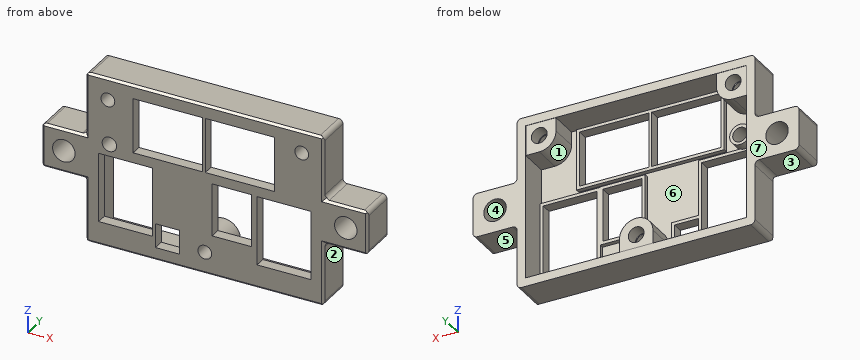
```python
from build123d import *

# Parameters (mm, degrees)
SKETCH1_W           = 54
SKETCH1_H           = 39
SKETCH1_W_2         = 10
SKETCH1_H_2         = 10
SKETCH1_R           = 2.5527
BOSS_EXTRUDE1_DEPTH = 8
SKETCH2_W           = 50.1
SKETCH2_H           = 35.1
CUT_EXTRUDE1_DEPTH  = 0.0762
CUT_EXTRUDE2_DEPTH  = 6.5
SKETCH4_R           = 1.56
CUT_EXTRUDE3_DEPTH  = 43.568023286
SKETCH5_R           = 1.79
CUT_EXTRUDE4_DEPTH  = 2.92
SKETCH6_W           = 12.25
SKETCH6_H           = 15.75
SKETCH6_W_2         = 15.75
SKETCH6_H_2         = 12.5
SKETCH6_W_3         = 5.5
SKETCH6_H_3         = 5.5
CUT_EXTRUDE5_DEPTH  = 43.337883821
SKETCH7_W           = 8.9
SKETCH7_H           = 12
CUT_EXTRUDE6_DEPTH  = 43.337883821
CHAMFER1_SIZE       = 0.5
SKETCH9_R           = 1.651
CUT_EXTRUDE8_DEPTH  = 43.337883821
BOSS_EXTRUDE2_START = 3
SKETCH10_R          = 2.3375
SKETCH10_R_2        = 1.651
BOSS_EXTRUDE2_DEPTH = 3
SKETCH11_W          = 5.5
SKETCH11_H          = 5.5
SKETCH11_W_2        = 12.25
SKETCH11_H_2        = 15.75
SKETCH11_W_3        = 8.9
SKETCH11_H_3        = 12
SKETCH11_W_4        = 15.75
SKETCH11_H_4        = 12.5
BOSS_EXTRUDE3_DEPTH = 1
FILLET1_R           = 1


with BuildPart() as part:
    # Sketch1 → Boss-Extrude1 (new body)
    # profile 1 of 3: a face of its own
    with BuildSketch(Plane(origin=(0, 0, 0), x_dir=(1, 0, 0), z_dir=(0, 1, 0))):
        Rectangle(SKETCH1_W, SKETCH1_H)
    # profile 2 of 3: a face of its own
    with BuildSketch(Plane(origin=(0, 0, 0), x_dir=(1, 0, 0), z_dir=(0, 1, 0))):
        with Locations((32, 0)):
            Rectangle(SKETCH1_W_2, SKETCH1_H_2)
        with Locations(Location((32, 0, 0), (0, 0, 270))):
            Circle(SKETCH1_R, mode=Mode.SUBTRACT)
    # profile 3 of 3: a face of its own
    with BuildSketch(Plane(origin=(0, 0, 0), x_dir=(1, 0, 0), z_dir=(0, 1, 0))):
        with Locations((-32, 0)):
            Rectangle(SKETCH1_W_2, SKETCH1_H_2)
        with Locations(Location((-32, 0, 0), (0, 0, 270))):
            Circle(SKETCH1_R, mode=Mode.SUBTRACT)
    extrude(amount=BOSS_EXTRUDE1_DEPTH)

    # Sketch2 → Cut-Extrude1 (cut)
    with BuildSketch(Plane(origin=(0, 8, 0), x_dir=(1, 0, 0), z_dir=(0, 1, 0))):
        Rectangle(SKETCH2_W, SKETCH2_H)
    extrude(amount=-CUT_EXTRUDE1_DEPTH, mode=Mode.SUBTRACT)

    # Sketch3 → Cut-Extrude2 (cut)
    with BuildSketch(Plane(origin=(0, 7.9238, 0), x_dir=(1, 0, 0), z_dir=(0, 1, 0))):
        with BuildLine():
            Line((-3.79, 14.5), (-3.79, 17.55))
            Line((-3.79, 17.55), (-25.05, 17.55))
            Line((-25.05, 17.55), (-25.05, -10.71))
            Line((-25.05, -10.71), (-22, -10.71))
            ThreePointArc((-22, -10.71), (-19.320065299, -11.820065299), (-18.21, -14.5))
            Line((-18.21, -14.5), (-18.21, -17.55))
            Line((-18.21, -17.55), (18.21, -17.55))
            Line((18.21, -17.55), (18.21, -14.5))
            ThreePointArc((18.21, -14.5), (19.320065299, -11.820065299), (22, -10.71))
            Line((22, -10.71), (25.05, -10.71))
            Line((25.05, -10.71), (25.05, 17.55))
            Line((25.05, 17.55), (3.79, 17.55))
            Line((3.79, 17.55), (3.79, 14.5))
            ThreePointArc((3.79, 14.5), (0, 10.71), (-3.79, 14.5))
        make_face()
    extrude(amount=-CUT_EXTRUDE2_DEPTH, mode=Mode.SUBTRACT)

    # Sketch4 → Cut-Extrude3 (cut, through all)
    with BuildSketch(Plane(origin=(0, 7.9238, 0), x_dir=(1, 0, 0), z_dir=(0, 1, 0))):
        with Locations(Location((0, 14.5, 0), (0, 0, 270))):
            Circle(SKETCH4_R)
        with Locations(Location((-22, -14.5, 0), (0, 0, 270))):
            Circle(SKETCH4_R)
        with Locations(Location((22, -14.5, 0), (0, 0, 90))):
            Circle(SKETCH4_R)
    extrude(amount=-CUT_EXTRUDE3_DEPTH, mode=Mode.SUBTRACT)

    # Sketch5 → Cut-Extrude4 (cut)
    with BuildSketch(Plane(origin=(0, 7.9238, 0), x_dir=(1, 0, 0), z_dir=(0, 1, 0))):
        with Locations(Location((0, 14.5, 0), (0, 0, 270))):
            Circle(SKETCH5_R)
        with Locations(Location((-22, -14.5, 0), (0, 0, 270))):
            Circle(SKETCH5_R)
        with Locations(Location((22, -14.5, 0), (0, 0, 90))):
            Circle(SKETCH5_R)
    extrude(amount=-CUT_EXTRUDE4_DEPTH, mode=Mode.SUBTRACT)

    # Sketch6 → Cut-Extrude5 (cut, through all)
    with BuildSketch(Plane(origin=(0, 1.4238, 0), x_dir=(1, 0, 0), z_dir=(0, 1, 0))):
        with Locations((17.975, 6.255)):
            Rectangle(SKETCH6_W, SKETCH6_H)
        with Locations((7.975, -10.15)):
            Rectangle(SKETCH6_W_2, SKETCH6_H_2)
        with Locations((-17.975, 6.255)):
            Rectangle(SKETCH6_W, SKETCH6_H)
        with Locations((-8.4, -10.15)):
            Rectangle(SKETCH6_W_2, SKETCH6_H_2)
        with Locations((-8.45, 13.8)):
            Rectangle(SKETCH6_W_3, SKETCH6_H_3)
    extrude(amount=-CUT_EXTRUDE5_DEPTH, mode=Mode.SUBTRACT)

    # Sketch7 → Cut-Extrude6 (cut, through all)
    with BuildSketch(Plane(origin=(0, 1.4238, 0), x_dir=(1, 0, 0), z_dir=(0, 1, 0))):
        with Locations((6.1, 4.28)):
            Rectangle(SKETCH7_W, SKETCH7_H)
    extrude(amount=-CUT_EXTRUDE6_DEPTH, mode=Mode.SUBTRACT)

    # Chamfer1
    chamfer1_edges = [part.edges().sort_by_distance(p)[0] for p in [
        (-27, 0, 12.25),
        (-32, 0, 5),
        (-37, 0, 0),
        (-32, 0, -5),
        (-27, 0, -12.25),
        (0, 0, -19.5),
        (27, 0, -12.25),
        (32, 0, -5),
        (37, 0, 0),
        (32, 0, 5),
        (27, 0, 12.25),
        (0, 0, 19.5),
    ]]
    chamfer(chamfer1_edges, length=CHAMFER1_SIZE)

    # Sketch9 → Cut-Extrude8 (cut, through all)
    with BuildSketch(Plane(origin=(0, 1.4238, 0), x_dir=(1, 0, 0), z_dir=(0, 1, 0))):
        with Locations(Location((-21.65, -4.35, 0), (0, 0, 270))):
            Circle(SKETCH9_R)
    extrude(amount=-CUT_EXTRUDE8_DEPTH, mode=Mode.SUBTRACT)

    # Sketch10 → Boss-Extrude2 (add)
    with BuildSketch(Plane(origin=(0, 1.4238, 0), x_dir=(1, 0, 0), z_dir=(0, 1, 0)).offset(BOSS_EXTRUDE2_START)):
        with Locations(Location((-21.65, -4.406538836, 0), (0, 0, 270))):
            Circle(SKETCH10_R)
        with Locations(Location((-21.65, -4.35, 0), (0, 0, 270))):
            Circle(SKETCH10_R_2, mode=Mode.SUBTRACT)
    extrude(amount=-BOSS_EXTRUDE2_DEPTH)

    # Sketch11 → Boss-Extrude3 (add)
    # profile 1 of 3: a face of its own
    with BuildSketch(Plane(origin=(0, 1.4238, 0), x_dir=(1, 0, 0), z_dir=(0, 1, 0))):
        Polygon((-11.15, -2.32), (-11.15, 10.35), (-5, 10.35), (-5, 17.25), (-11.9, 17.25), (-11.9, 14.83), (-24.8, 14.83), (-24.8, -2.32), align=None)
        with Locations((-8.45, 13.8)):
            Rectangle(SKETCH11_W, SKETCH11_H, mode=Mode.SUBTRACT)
        with Locations((-17.975, 6.255)):
            Rectangle(SKETCH11_W_2, SKETCH11_H_2, mode=Mode.SUBTRACT)
    # profile 2 of 3: a face of its own
    with BuildSketch(Plane(origin=(0, 1.4238, 0), x_dir=(1, 0, 0), z_dir=(0, 1, 0))):
        Polygon((0.95, 10.98), (0.95, -2.42), (11.25, -2.42), (11.25, -2.32), (24.8, -2.32), (24.8, 14.83), (11.15, 14.83), (11.15, 10.98), align=None)
        with Locations((17.975, 6.255)):
            Rectangle(SKETCH11_W_2, SKETCH11_H_2, mode=Mode.SUBTRACT)
        with Locations((6.1, 4.28)):
            Rectangle(SKETCH11_W_3, SKETCH11_H_3, mode=Mode.SUBTRACT)
    # profile 3 of 3: a face of its own
    with BuildSketch(Plane(origin=(0, 1.4238, 0), x_dir=(1, 0, 0), z_dir=(0, 1, 0))):
        Polygon((16.55, -3.2), (0.175, -3.2), (-16.975, -3.2), (-16.975, -17.1), (0.175, -17.1), (16.55, -17.1), align=None)
        with Locations((7.975, -10.15)):
            Rectangle(SKETCH11_W_4, SKETCH11_H_4, mode=Mode.SUBTRACT)
        with Locations((-8.4, -10.15)):
            Rectangle(SKETCH11_W_4, SKETCH11_H_4, mode=Mode.SUBTRACT)
    extrude(amount=BOSS_EXTRUDE3_DEPTH)

    # Fillet1
    fillet1_edges = [part.edges().sort_by_distance(p)[0] for p in [
        (-27, 4.25, 19.5),
        (-27, 4.25, 5),
        (-37, 4.25, 5),
        (-37, 4.25, -5),
        (-27, 4.25, -5),
        (-27, 4.25, -19.5),
        (27, 4.25, -19.5),
        (27, 4.25, -5),
        (37, 4.25, -5),
        (37, 4.25, 5),
        (27, 4.25, 5),
        (27, 4.25, 19.5),
    ]]
    fillet(fillet1_edges, radius=FILLET1_R)


solid = part.part
```
Check sheet for the modelled part. Datum: model origin and axes. Units: mm. Face numbers are marked on the shaded views. A direction names the side the tool comes from. Round coordinates to 2 decimals unless told otherwise and drop trailing zeros. Write each loop counter-clockwise with the first axis right and the second up, starting at its lowest first coordinate (ties: lowest second). Pieces come first, ordered by that corner, then holes. Notation, with made-up numbers: (24, 57.5) -> (46, 57.5) arc R17 ccw to (46, 64.5) -> close; hole circle Ø5 at (-39.75, -6). An arc over 180 degrees is marked (long way). One line per question, with ' | ' between items. Start each with the question number.
1. Sectioned sample at D-D, the plane x = -32. Record the cut outline in (y, z), then the cut area to 3 significant figures.
2. Set-up check for the marked faces 1, 2 and 3: record each of +Z, -Z, +X, -X, +Y, -Y from which the full face is reachable in a straight line by a thin tool's end or side.
3. Depth check by flat-ended pin: pin 1 (2 mm diameter, centred on y = 2, z = 14.5, fed in from -X); pin 2 (3 mm diameter, centred on y = 4.5, z = 9, fed in from +X); pin 3 (5.5 mm diameter, centred on x = 21, z = 13, fed in from +Y). Enter the tip coordinate at first touch or a pass-through.
4. Release check for a two-part mould opening along Z. For the marked faces 4, 5, 6 and 7 record: +Z half, -Z half, draft (parallel to the pull), parting line (faces both ways), or undercut.
5. Scan lines: line 1 along X through (y, z) = (1.25, -7); line 2 along X through (y, z) = (6.65, -14.5); line 3 along Z through (x, y) = (-11, 1). Record each from-to range of solid material in increasing order. Write a range as from..to.
6. Sectioned sample at A-A, the plane x = -8. Record the cut outline in (y, z).
7. Sectioned sample at B-B, the plane z = 9. Record the cut outline in (x, y) (3 decimals), then the cut area to 3 significant figures.
8. Sectioned sample at C-C, the plane y = 3.5. Count the separate pieces of the cut face and the enclosed holes in it, then the cut area to 3 significant figures.
Taken from the geometry:
1) outline: (0, -4.5) -> (0.5, -5) -> (8, -5) -> (8, -2.55) -> (0, -2.55) -> close; (0, 2.55) -> (8, 2.55) -> (8, 5) -> (0.5, 5) -> (0, 4.5) -> close | area: 38.9 mm^2
2) face 1: +Y | face 2: -Z, +X, +Y, -Y | face 3: -Z, -X, +Y, -Y
3) pin 1: stops at x = -27 | pin 2: stops at x = 27 | pin 3: stops at y = 7.92
4) face 4: undercut | face 5: -Z half | face 6: undercut | face 7: draft
5) line 1: x = -27..-24.1, -11.85..1.65, 10.55..11.85, 24.1..27 | line 2: x = -27..-25.05, -3.79..-1.79, 1.79..3.79, 25.05..27 | line 3: z = -19.5..-16.55, -11.05..3.9, 16.4..19.5
6) outline: (0, -19) -> (0.5, -19.5) -> (8, -19.5) -> (8, -17.55) -> (1.42, -17.55) -> (1.42, -17.25) -> (2.42, -17.25) -> (2.42, -16.55) -> (0, -16.55) -> close; (0, -11.05) -> (2.42, -11.05) -> (2.42, -10.35) -> (1.42, -10.35) -> (1.42, 3.2) -> (2.42, 3.2) -> (2.42, 3.9) -> (0, 3.9) -> close; (0, 16.4) -> (2.42, 16.4) -> (2.42, 17.1) -> (1.42, 17.1) -> (1.42, 17.55) -> (8, 17.55) -> (8, 19.5) -> (0.5, 19.5) -> (0, 19) -> close
7) outline: (-27, 0.5) -> (-26.5, 0) -> (-16.275, 0) -> (-16.275, 2.424) -> (-16.975, 2.424) -> (-16.975, 1.424) -> (-25.05, 1.424) -> (-25.05, 8) -> (-27, 8) -> close; (-0.525, 0) -> (0.1, 0) -> (0.1, 2.424) -> (-0.525, 2.424) -> close; (15.85, 0) -> (26.5, 0) -> (27, 0.5) -> (27, 8) -> (25.05, 8) -> (25.05, 1.424) -> (16.55, 1.424) -> (16.55, 2.424) -> (15.85, 2.424) -> close | area: 59.5 mm^2
8) separate pieces: 2 | enclosed holes: 7 | area: 624 mm^2
